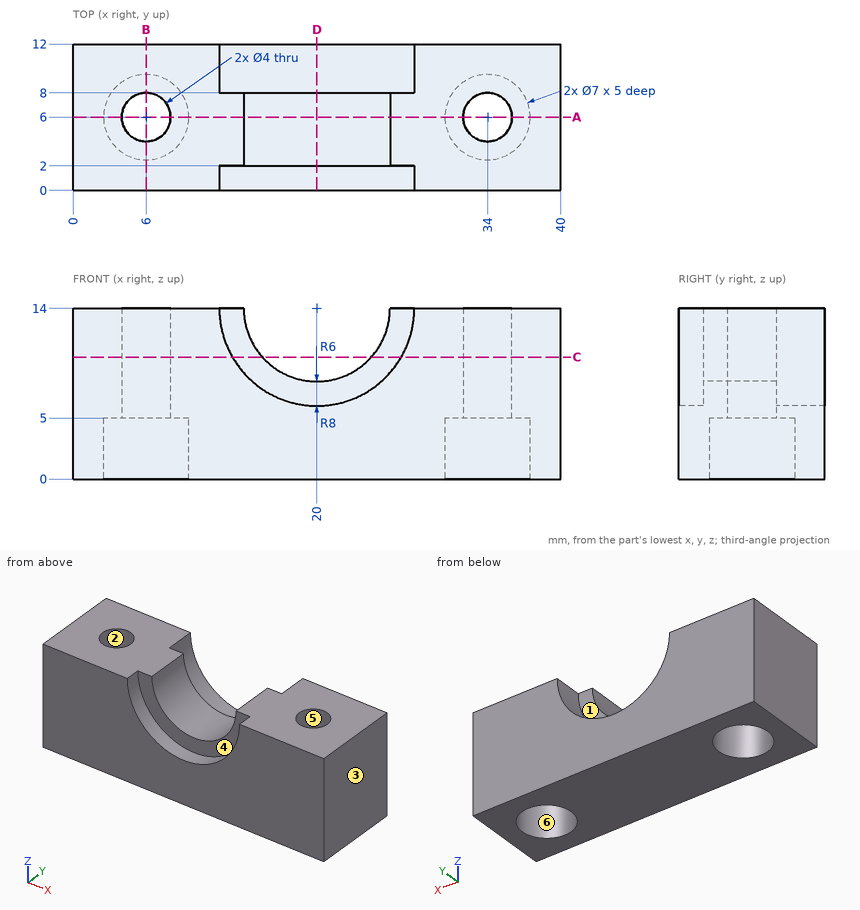
Can you work these out from the drawing? Everything is in mm from the part's minimum corner. A direction names the side the tool comes from. Coordinates: 2 decimals unless noted, no trailing zeros. Order: outer loops, then holes, each group sorted by start corner. A loop starts at its lowest first (then second) coordinate and runs counter-clockwise, first axis right, second up. Notation, with made-up numbers: (12, 10.25) -> (24, 10.25) arc R13 cw to (24, 23.25) -> close; hole circle Ø2 at (-8, 16). An arc over 180 degrees is marked (long way). Return JSON: item names as keys, results as strings.
1) I'm going to push a flat-ended pin straight in: P1, Ø5, axis at x = 34, y = 6, coming from the -Z side. Where does the tip first touch, or does it pass through?
Conclusion:
{"P1": "stops at z = 5"}
2) If we section it at C-C on z = 10: List the corners of the cut face in (x, y) for me.
Conclusion:
{"outline": "(0, 0) -> (13.07, 0) -> (13.07, 2) -> (15.53, 2) -> (15.53, 8) -> (13.07, 8) -> (13.07, 12) -> (0, 12) -> close; (24.47, 2) -> (26.93, 2) -> (26.93, 0) -> (40, 0) -> (40, 12) -> (26.93, 12) -> (26.93, 8) -> (24.47, 8) -> close; hole circle Ø4 at (6, 6); hole circle Ø4 at (34, 6)"}
3) If we section it at A-A on y = 6: List the corners of the cut face in (x, z) for me, plus the area to 3 significant figures.
Conclusion:
{"outline": "(0, 0) -> (2.5, 0) -> (2.5, 5) -> (4, 5) -> (4, 14) -> (0, 14) -> close; (8, 5) -> (9.5, 5) -> (9.5, 0) -> (30.5, 0) -> (30.5, 5) -> (32, 5) -> (32, 14) -> (26, 14) arc R6 cw to (14, 14) -> (8, 14) -> close; (36, 5) -> (37.5, 5) -> (37.5, 0) -> (40, 0) -> (40, 14) -> (36, 14) -> close", "area": "361 mm²"}
4) If we section it at D-D on x = 20: List the corners of the cut face in (y, z) for me, plus the area to 3 significant figures.
Conclusion:
{"outline": "(0, 0) -> (12, 0) -> (12, 6) -> (8, 6) -> (8, 8) -> (2, 8) -> (2, 6) -> (0, 6) -> close", "area": "84.0 mm²"}
5) If I drill on probe 1 along X at (y, z) = (6, 7.75); probe 2 along Y at (x, z) = (6, 2.75); probe 3 along X at (y, z) = (7.25, 4.5), over which ranges is the centre line in solid material (lowest first)?
Conclusion:
{"probe 1": "x = 0 to 4, 8 to 32, 36 to 40", "probe 2": "y = 0 to 2.5, 9.5 to 12", "probe 3": "x = 0 to 2.73, 9.27 to 30.73, 37.27 to 40"}
6) If we section it at B-B on x = 6: List the corners of the cut face in (y, z) for me.
Conclusion:
{"outline": "(0, 0) -> (2.5, 0) -> (2.5, 5) -> (4, 5) -> (4, 14) -> (0, 14) -> close; (8, 5) -> (9.5, 5) -> (9.5, 0) -> (12, 0) -> (12, 14) -> (8, 14) -> close"}
7) Thinking about a two-plate mould opening in Y: for the marked faces 1, 2 and 3, which applies, +Y half, -Y half, draft (parallel to the pull), parting line (faces both ways), or undercut?
Conclusion:
{"face 1": "+Y half", "face 2": "undercut", "face 3": "draft"}
8) On a 3-axis mill with a long thin cutter (end or side, diameter ignored), from which of +Z, -Z, +X, -X, +Y, -Y can I reach the whole of each face in a straight line? I mean the marked faces 4, 5 and 6. Say none if no direction works.
Conclusion:
{"face 4": "+Z, -Y", "face 5": "+Z, -Z", "face 6": "-Z"}
